The listing builds one solid part. Answer for the finished solid, in the listing's coordinates (mm). A direction names the side the tool comes from. Coordinates: 2 decimals unless noted, no trailing zeros. Order: outer loops, then holes, each group sorted by start corner. A loop starts at its lowest first (then second) coordinate and runs counter-clockwise, first axis right, second up. Notation, with made-up numbers: (-37, 3.5) -> (-13, 3.5) arc R24 ccw to (-13, 27.5) -> close; hole circle Ø7 at (59.5, -0.75). An arc over 180 degrees is marked (long way). Answer in a Markdown table with one row per item. Add a question column.
```python
from build123d import *

# Parameters (mm, degrees)
F0_W        = 76.2
F0_H        = 38.1
F1_DEPTH    = 7.62
F4_DEPTH    = 7.621
F6_DEPTH    = 38.101
F7_T4_DEPTH = 38.1
F8_T4_DEPTH = 42.4215480701
F9_R        = 5.08


# Not quite as in the source:
# - a fillet or chamfer that OpenCascade refuses, or shapes differently, is made with other operations: its cross-section is extruded or revolved along the edge and cut away or added
# - a feature names something its author has since deleted; it is built from what else it names


with BuildPart() as f1:
    # F0 (on Top) → F1 (new body)
    with BuildSketch(Plane.XY):
        Rectangle(F0_W, F0_H)
    extrude(amount=F1_DEPTH)

    # F3 (on face) → F4 (cut, through all)
    with BuildSketch(Plane.XY.offset(7.62)):
        Polygon((-38.1, -6.35), (-38.1, -19.05), (-20.32, -19.05), (20.32, -19.05), align=None)
    extrude(amount=-F4_DEPTH, mode=Mode.SUBTRACT)

    # F5 (on face) → F6 (cut, through all)
    with BuildSketch(Plane(origin=(0, 19.05, 0), x_dir=(-1, 0, 0), z_dir=(0, 1, 0))):
        Polygon((38.1, 7.62), (-20.32, 7.62), (-20.32, 3.81), (20.32, 3.81), (20.32, 5.715), (38.1, 5.715), align=None)
    extrude(amount=-F6_DEPTH, mode=Mode.SUBTRACT)

    # F7: chamfer of 7.62 x 5.08 on 1 edges, made by hand


with BuildPart() as f7_tool2:
    # F7_s3 → F7_t4 (new body)
    with BuildSketch(Plane.XZ.offset(-19.05)):
        Polygon((20.32, 8.89), (12.7, 3.81), (20.32, 3.81), align=None)
    extrude(amount=F7_T4_DEPTH)

    split(bisect_by=Plane.XY.offset(7.62), keep=Keep.BOTTOM)

    split(bisect_by=Plane(origin=(-3.0374548736, -13.9722924188, 0), x_dir=(0, 0, 1), z_dir=(0.2124296443, 0.9771763639, 0)), keep=Keep.TOP)


with BuildPart() as f1_1:
    add(f1.part)

    # F7_t1: union F7_tool2
    add(f7_tool2.part)

    # F8: chamfer of 2.54 x 5.08 on 1 edges, made by hand


with BuildPart() as f8_tool2:
    # F8_s3 → F8_t4 (new body)
    with BuildSketch(Plane.XZ.offset(-19.05)):
        Polygon((-20.32, 6.35), (-15.24, 3.81), (-20.32, 3.81), align=None)
    extrude(amount=F8_T4_DEPTH)

    split(bisect_by=Plane.XY.offset(5.715), keep=Keep.BOTTOM)

    split(bisect_by=Plane(origin=(-3.0374548736, -13.9722924188, 0), x_dir=(0, 0, 1), z_dir=(0.2124296443, 0.9771763639, 0)), keep=Keep.TOP)


with BuildPart() as f1_2:
    add(f1_1.part)

    # F8_t1: union F8_tool2
    add(f8_tool2.part)

    # F9
    f9_edges = [f1_2.edges().sort_by_distance(p)[0] for p in [
        (-38.1, -6.35, 2.8575),
        (-38.1, 19.05, 2.8575),
        (38.1, -19.05, 3.81),
        (38.1, 19.05, 3.81),
    ]]
    fillet(f9_edges, radius=F9_R)


solid = f1_2.part
```
Q1. Straight lines are drawn through the part: line 1 (Z direction, x = 3, y = -14.5); line 2 (Z direction, x = -22, y = -1.5) (3 decimals); line 3 (X direction, y = 1.5, z = 4.5) (3 decimals). For each, find the intervals that lie inside material, in ascending order.
Q2. A cutting plane is placed at B-B (z = 4.5). Determine the outline of the cut face in (x, y) (3 decimals).
Q3. A cutting plane is placed at D-D (x = -6). Determine the outline of the cut face in (y, z), then the cut area to 3 significant figures.
Q4. Determine the mould class of faces 3 (the face through (36.572, -17.601, 3.863)), 4 (the face through (-29, 4, 5.715)), 5 (the face through (15.598, 0.471, 5.742)) for opening direction X: +X half, -X half, draft (parallel to the pull), parting line (faces both ways), or undercut.
Q5. For faces 1 (the face through (28, 0, 7.62)), 2 (the face through (-1, 1, 3.81)), determine the directions among +Z, -Z, +X, -X, +Y, -Y from which every point of the face is accessible in a straight line to the end or side of a thin tool.
Q6. A cutting plane is placed at C-C (y = 10). Determine the outline of the cut face in (x, z) (3 decimals).
Q7. Given pin 1 (8.5 mm diameter, centred on x = 2.5, y = -5, fed in from +Z); pin 2 (2 mm diameter, centred on y = -4.5, z = 1, fed in from -X); pin 3 (5.5 mm diameter, centred on x = -27, y = 10, fed in from +Z) (3 decimals), each flat-ended and moving along its own axis, determine where each tip first touches the part or whether it passes through.
Q8. A cutting plane is placed at A-A (z = 1). Determine the outline of the cut face in (x, y).
Returned:
| question | item | result |
|---|---|---|
| 1 | line 1 | z = 0 to 3.81 |
| 1 | line 2 | z = 0 to 5.715 |
| 1 | line 3 | x = -38.1 to -16.62, 13.735 to 38.1 |
| 2 | outline | (-38.1, -2.256) arc R5.08 ccw to (-34.099, -7.22) -> (-16.62, -11.02) -> (-16.62, 19.05) -> (-33.02, 19.05) arc R5.08 ccw to (-38.1, 13.97) -> close; (13.735, -17.618) -> (20.32, -19.05) -> (33.02, -19.05) arc R5.08 ccw to (38.1, -13.97) -> (38.1, 13.97) arc R5.08 ccw to (33.02, 19.05) -> (13.735, 19.05) -> close |
| 3 | outline | (-13.33, 0) -> (19.05, 0) -> (19.05, 3.81) -> (-13.33, 3.81) -> close |
| 3 | area | 123 mm² |
| 4 | face 3 | +X half |
| 4 | face 4 | draft |
| 4 | face 5 | undercut |
| 5 | face 1 | +Z, +X, -X, +Y, -Y |
| 5 | face 2 | +Z, +Y, -Y |
| 6 | outline | (-38.1, 0) -> (38.1, 0) -> (38.1, 7.62) -> (18.415, 7.62) -> (12.7, 3.81) -> (-15.24, 3.81) -> (-19.05, 5.715) -> (-38.1, 5.715) -> close |
| 7 | pin 1 | stops at z = 3.81 |
| 7 | pin 2 | stops at x = -37.95 |
| 7 | pin 3 | stops at z = 5.715 |
| 8 | outline | (-38.1, -2.26) arc R5.08 ccw to (-34.1, -7.22) -> (20.32, -19.05) -> (33.02, -19.05) arc R5.08 ccw to (38.1, -13.97) -> (38.1, 13.97) arc R5.08 ccw to (33.02, 19.05) -> (-33.02, 19.05) arc R5.08 ccw to (-38.1, 13.97) -> close |
